Verification items for the finished model (mm, model axes). A direction names the side the tool comes from. Give positions to 0.01 mm unless a question says otherwise; leave off trailing zeros. Order: outer loops, then holes, each group sorted by start corner. A loop starts at its lowest first (then second) coordinate and runs counter-clockwise, first axis right, second up.
from build123d import *

# Parameters (mm, degrees)
F1_DEPTH             = 5
F4_D                 = 3.2
F4_CBORE_D           = 6.2
F4_CBORE_DEPTH       = 2
F4_ON_F3_D           = 3.2
F4_ON_F3_CBORE_D     = 6.2
F4_ON_F3_CBORE_DEPTH = 2
F5_R                 = 1
F6_T1_DEPTH          = 25


# Not quite as in the source:
# - a fillet or chamfer that OpenCascade refuses, or shapes differently, is made with other operations: its cross-section is extruded or revolved along the edge and cut away or added


with BuildPart() as f1:
    # F0 (on Front) → F1 (new body, symmetric)
    with BuildSketch(Plane.XZ):
        Polygon((0, 74), (0, 0), (4, 0), (4, 70), (14, 70), (14, 74), align=None)
    extrude(amount=F1_DEPTH, both=True)

    # F4 (through all)
    with Locations(Plane(origin=(0, 0, 0), x_dir=(0, -1, 0), z_dir=(-1, 0, 0))):
        with Locations((0, 24), (0, 4)):
            CounterBoreHole(F4_D / 2, F4_CBORE_D / 2, F4_CBORE_DEPTH)

    # F4 on F3 (through all)
    with Locations(Plane(origin=(0, 0, 70), x_dir=(1, 0, 0), z_dir=(0, 0, -1))):
        with Locations((9, 0)):
            CounterBoreHole(F4_ON_F3_D / 2, F4_ON_F3_CBORE_D / 2, F4_ON_F3_CBORE_DEPTH)

    # F5
    f5_edges = [f1.edges().sort_by_distance(p)[0] for p in [
        (4, 0, 70),
    ]]
    fillet(f5_edges, radius=F5_R)

    # F6: fillet of radius 3 on 1 edges, made by hand

    # F6_s2 → F6_t1 (cut)
    with BuildSketch(Plane.XZ.offset(-12.5)):
        with BuildLine():
            ThreePointArc((3, 0), (0.8786796564, 0.8786796564), (0, 3))
            Line((0, 3), (0, 0))
            Line((0, 0), (3, 0))
        make_face()
    extrude(amount=F6_T1_DEPTH, mode=Mode.SUBTRACT)


solid = f1.part
(1) Release check for a two-part mould opening along Y. For faces 1 (the cylindrical face through (0.986, 0.672, 20.974)), 2 (the flat face through (3.8, -5, 45.7)), 3 (the flat face through (12.4, -0.1, 70)) record: pulls with the +Y half, pulls with the -Y half, needs draft (parallel to the pull), parting line crosses it, or undercut.
Solved:
face 1: undercut
face 2: pulls with the -Y half
face 3: needs draft
(2) Section check A-A, the plane x = 9. Enter the section's corners in (y, z), then the cut area to 3 significant figures.
Solved:
outline: (-5, 70) - (-3.1, 70) - (-3.1, 72) - (-1.6, 72) - (-1.6, 74) - (-5, 74) - close; (1.6, 72) - (3.1, 72) - (3.1, 70) - (5, 70) - (5, 74) - (1.6, 74) - close
area: 21.2 mm2
(3) Set-up check for faces 4 (the flat face through (4, 0, 34)), 5 (the cylindrical face through (5.9, -0.1, 71)), 6 (the flat face through (2, -1.3, 2.7)), 7 (the flat face through (0, 0, 39)): record each of +Z, -Z, +X, -X, +Y, -Y from which the full face is reachable in a straight line by a thin tool's end or side.
Solved:
face 4: -Z, +X, +Y, -Y
face 5: -Z
face 6: -X
face 7: +Z, -Z, -X, +Y, -Y
(4) Section check B-B, the plane z = 24. Enter the section's corners in (x, y), then the cut area to 3 significant figures.
Solved:
outline: (0, -5) - (4, -5) - (4, -1.6) - (2, -1.6) - (2, -3.1) - (0, -3.1) - close; (0, 3.1) - (2, 3.1) - (2, 1.6) - (4, 1.6) - (4, 5) - (0, 5) - close
area: 21.2 mm2
(5) Section check D-D, the plane y = 0. Give the number of separate pieces and of enclosed holes in the cut face, then the cut area to 3 significant figures.
Solved:
separate pieces: 4
enclosed holes: 0
area: 278 mm2
(6) Section check C-C, the plane y = -4.25. Enter the section's corners in (x, z), then the cut area to 3 significant figures.
Solved:
outline: (0, 3) arc R3 ccw to (3, 0) - (4, 0) - (4, 69) arc R1 cw to (5, 70) - (14, 70) - (14, 74) - (0, 74) - close
area: 334 mm2
(7) Go/stop test with flat-tipped pins: pin 1 (8 mm diameter, centred on x = 6, z = 16, fed in from -Y); pin 2 (1.9 mm diameter, centred on y = 1, z = 24.5, fed in from -X); pin 3 (5 mm diameter, centred on x = 9, y = 0, fed in from -Z); pin 4 (6 mm diameter, centred on y = 1.5, z = 40.5, fed in from +X). Record where each tip stops, or that it passes through.
Solved:
pin 1: stops at y = -5
pin 2: stops at x = 2
pin 3: stops at z = 72
pin 4: stops at x = 4
(8) Scan lines: line 1 (Z direction, x = 1.5, y = 2.5); line 2 (Z direction, x = 2.5, y = 0.5); line 3 (Z direction, x = 12.75, y = -2). Record each from-to range of solid material in increasing order.
Solved:
line 1: z = 0.4 to 2.17, 5.83 to 22.17, 25.83 to 74
line 2: z = 0.04 to 2.48, 5.52 to 22.48, 25.52 to 74
line 3: z = 70 to 74
